Source: CAD feature listing. Evaluate the final solid. Frame: model axes, mm. Coordinates: 2 decimals unless noted, no trailing zeros. Order: outer loops, then holes, each group sorted by start corner. A loop starts at its lowest first (then second) coordinate and runs counter-clockwise, first axis right, second up. Notation, with made-up numbers: (-38, 64.25) -> (20, 64.25) arc R19 cw to (20, 86.25) -> close; hole circle Ø2 at (69, 4). An arc over 180 degrees is marked (long way). Put each result on its own line as item: value.
from build123d import *

# Parameters (mm, degrees)
SKETCH1_W           = 127
SKETCH1_H           = 50.8
SKETCH1_R           = 3.2639
BOSS_EXTRUDE1_DEPTH = 3.175
SKETCH2_R           = 14.2875
CUT_EXTRUDE1_DEPTH  = 137.930502446


with BuildPart() as part:
    # Sketch1 → Boss-Extrude1 (new, symmetric)
    with BuildSketch(Plane.XY):
        with Locations((63.5, 25.4)):
            Rectangle(SKETCH1_W, SKETCH1_H)
        with Locations((88.9, 12.7)):
            Circle(SKETCH1_R, mode=Mode.SUBTRACT)
        with Locations((114.3, 12.7)):
            Circle(SKETCH1_R, mode=Mode.SUBTRACT)
        with Locations((88.9, 38.1)):
            Circle(SKETCH1_R, mode=Mode.SUBTRACT)
        with Locations((114.3, 38.1)):
            Circle(SKETCH1_R, mode=Mode.SUBTRACT)
    extrude(amount=BOSS_EXTRUDE1_DEPTH, both=True)

    # Sketch2 → Cut-Extrude1 (cut, through all)
    with BuildSketch(Plane.XY.offset(3.175)):
        with Locations((31.75, 25.4)):
            Circle(SKETCH2_R)
    extrude(amount=-CUT_EXTRUDE1_DEPTH, mode=Mode.SUBTRACT)


solid = part.part
1. Pull-direction query (X, two-part tool) for faces 1 (the cylindrical face through (45.38, 29.69, 0.04)), 2 (the flat face through (63, 26, -3.175)), 3 (the cylindrical face through (117.413, 39.08, -0.044)), 4 (the flat face through (0, 25, 0)); classes: pulls with the +X half, pulls with the -X half, needs draft (parallel to the pull), parting line crosses it, or undercut.
Numbers:
face 1: undercut
face 2: needs draft
face 3: undercut
face 4: pulls with the -X half
2. Cut plane C-C on z = -1.75. Count the separate pieces of the cut face and the enclosed holes in it, plus the area to 3 significant figures.
Numbers:
separate pieces: 1
enclosed holes: 5
area: 5,680 mm2
3. First-contact query: pin 1 (4 mm diameter, centred on x = 114.3, y = 38.1, fed in from -Z); pin 2 (7.5 mm diameter, centred on x = 114.3, y = 12.7, fed in from +Z) (3 decimals). Flat tips, straight axial feed; report the tip coordinate or a pass-through.
Numbers:
pin 1: passes through
pin 2: stops at z = 3.175
4. Cut plane B-B on y = 25.4. Output: boundary loops of the cut face in (x, z) (1 decimal), plus the area to 3 significant figures.
Numbers:
outline: (0, -3.2) -> (17.5, -3.2) -> (17.5, 3.2) -> (0, 3.2) -> close; (46, -3.2) -> (127, -3.2) -> (127, 3.2) -> (46, 3.2) -> close
area: 625 mm2
5. Cut plane D-D on x = 114.3. Output: boundary loops of the cut face in (y, z) (3 decimals), plus the area to 3 significant figures.
Numbers:
outline: (0, -3.175) -> (9.436, -3.175) -> (9.436, 3.175) -> (0, 3.175) -> close; (15.964, -3.175) -> (34.836, -3.175) -> (34.836, 3.175) -> (15.964, 3.175) -> close; (41.364, -3.175) -> (50.8, -3.175) -> (50.8, 3.175) -> (41.364, 3.175) -> close
area: 240 mm2
6. Cut plane A-A on x = 31.75. Output: boundary loops of the cut face in (y, z) (1 decimal).
Numbers:
outline: (0, -3.2) -> (11.1, -3.2) -> (11.1, 3.2) -> (0, 3.2) -> close; (39.7, -3.2) -> (50.8, -3.2) -> (50.8, 3.2) -> (39.7, 3.2) -> close
7. Ray query, line 1 along Y through (x, z) = (88.9, -0.25); line 2 along Y through (x, z) = (42.5, -2); line 3 along X through (y, z) = (19, -1.5). Return the intervals inside material, ascending.
Numbers:
line 1: y = 0 to 9.44, 15.96 to 34.84, 41.36 to 50.8
line 2: y = 0 to 15.99, 34.81 to 50.8
line 3: x = 0 to 18.98, 44.52 to 127
